The model under review builds one solid part; all positions refer to its coordinate system, in mm. Face numbers are marked on the shaded views. A direction names the side the tool comes from. Round coordinates to 2 decimals unless told otherwise and drop trailing zeros. Write each loop counter-clockwise with the first axis right and the second up, starting at its lowest first coordinate (ties: lowest second). Pieces come first, ordered by that corner, then holes. Notation, with made-up numbers: (8.25, 37) -> (48.25, 37) arc R24 ccw to (48.25, 62) -> close; hole circle Ø8 at (-40, 65). An arc over 180 degrees is marked (long way). Use CSV: the item, a comma, the result in double quotes. Start each with the question number.
1) For pin 1 Ø3 at (y, z) = (2.5, -6.5) entering from -X; pin 2 Ø1.5 at (x, y) = (2, 1.5) entering from +Z; pin 3 Ø6 at (y, z) = (9, -5.5) entering from +X, all flat-tipped, find the tip position at first contact; note any pin that passes through.
2) Machinability: for the marked faces 4 and 5, which of the approach directions +Z, -Z, +X, -X, +Y, -Y give a long, thin tool a straight path to every point of the face, cutting with its end or side? Answer none if there is none.
3) Mouldability with a two-part tool opening along X and no side actions: class the marked faces 1, 2 and 3 as released by +X, released by -X, zero draft, split by the parting line, or undercut.
4) Take a section at C-C, the plane z = -2.75. Give the boundary of the cut face in (x, y).
5) Take a section at A-A, the plane z = 0. Give the boundary of the cut face in (x, y) (3 decimals).
6) Wall thickness on probe 1 along X at (y, z) = (7.5, 3.5); probe 2 along X at (y, z) = (2.25, -1.25); probe 3 along Z at (x, y) = (-3, 9.25): over which ranges is each line inside the solid? List them lowest first. Write a range as [from, to].
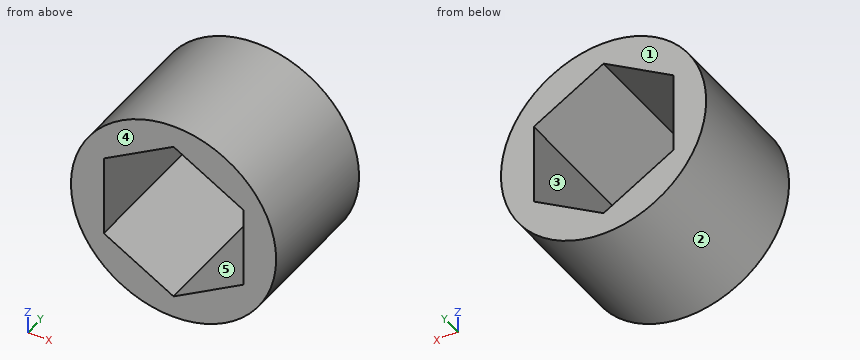
Autodesk Inventor part; units mm, degrees
ref_plane "YZ Plane" through (0, 0, 0) normal (1, 0, 0) x (0, 1, 0)
ref_plane "XZ Plane" through (0, 0, 0) normal (0, 1, 0) x (-1, 0, 0)
ref_plane "XY Plane" through (0, 0, 0) normal (0, 0, 1) x (1, 0, 0)
sketch "Sketch1" plane through (0, 0, 0) normal (0, 1, 0) x (-1, 0, 0)
  line L0 (0, -13.335) -> (0, 13.335)
  line L1 (-13.335, 0) -> (13.335, 0)
  circle A0 centre (0, 0) radius 9.525
  dimension "d0" = 19.05
extrude "Extrusion1" add sketch "Sketch1" along normal blind 12.7
sketch "Sketch2" plane through (0, 12.7, 0) normal (0, 1, 0) x (1, 0, 0)
  line L0 (0, 7.479) -> (6.477, 3.7395)
  line L1 (6.477, 3.7395) -> (6.477, -3.7395)
  line L2 (6.477, -3.7395) -> (0, -7.479)
  line L3 (0, -7.479) -> (-6.477, -3.7395)
  line L4 (-6.477, -3.7395) -> (-6.477, 3.7395)
  line L5 (-6.477, 3.7395) -> (0, 7.479)
  point P0 (0, 0)
  point P1 (0, 0)
  dimension "d3" = 12.954
extrude "Extrusion2" cut sketch "Sketch2" against normal through all
properties part number "ShaftSpacer0.5inHex"
Values found:
1,pin 1,"x = -8.11"
1,pin 2,"z = 9.44"
1,pin 3,"x = 9.19"
2,face 4,"+Z, -Z, +X, -X, -Y"
2,face 5,"+Y, -Y"
3,face 1,"zero draft"
3,face 2,"split by the parting line"
3,face 3,"undercut"
4,outline,"(-9.12, 0) -> (-6.48, 0) -> (-6.48, 12.7) -> (-9.12, 12.7) -> close; (6.48, 0) -> (9.12, 0) -> (9.12, 12.7) -> (6.48, 12.7) -> close"
5,outline,"(-9.525, 0) -> (-6.477, 0) -> (-6.477, 12.7) -> (-9.525, 12.7) -> close; (6.477, 0) -> (9.525, 0) -> (9.525, 12.7) -> (6.477, 12.7) -> close"
6,probe 1,"[-8.86, -6.48], [6.48, 8.86]"
6,probe 2,"[-9.44, -6.48], [6.48, 9.44]"
6,probe 3,"[-9.04, -5.75], [5.75, 9.04]"
